Autodesk Inventor part; units mm, degrees
ref_plane "YZ Plane" through (0, 0, 0) normal (1, 0, 0) x (0, 1, 0)
ref_plane "XZ Plane" through (0, 0, 0) normal (0, 1, 0) x (-1, 0, 0)
ref_plane "XY Plane" through (0, 0, 0) normal (0, 0, 1) x (1, 0, 0)
sketch "Эскиз1" plane through (0, 0, 0) normal (0, 0, 1) x (1, 0, 0)
  line L0 (-12.2268, 10) -> (34.5444, 10)
  line L1 (-55.4556, 0) -> (49.5444, 0)
  line L2 (-12.2268, -10) -> (34.5444, -10)
  arc A0 (-15.534, 11.25) -> (-15.534, -11.25) centre (-25.4556, 0) ccw
  circle A1 centre (-25.4556, 0) radius 5
  line L3 (34.5444, 10) -> (34.5444, -10)
  arc A2 (-15.534, 11.25) -> (-12.2268, 10) centre (-12.2268, 15) ccw
  arc A3 (-12.2268, -10) -> (-15.534, -11.25) centre (-12.2268, -15) ccw
  point P0 (0, 0)
  point P1 (-14.2752, 10)
  point P2 (-14.2752, -10)
  dimension "d0" = 15
  dimension "d1" = 20
  dimension "d2" = 10
  dimension "d12" = 5
  dimension "d13" = 60
extrude "Выдавливание1" add sketch "Эскиз1" along normal blind 5 and the other way blind 5 contours L0 L3 L1 A1 A0 A2 | L3 L2 A3 A0 L1 A1
sketch "Эскиз4" plane through (0, 0, 0) normal (0, 0, 1) x (1, 0, 0)
  line L0 (-20.9089, 0) -> (125.4533, 0)
  line L1 (34.5444, 10) -> (34.5444, -10)
  line L2 (34.5444, 0) -> (114.5444, 0)
  line L3 (114.5444, 0) -> (114.5444, 20)
  line L4 (114.5444, 20) -> (34.5444, 20)
  line L5 (34.5444, 20) -> (34.5444, 0)
  point P0 (0, 0)
  dimension "d7" = 40
  dimension "d8" = 80
revolve "Вращение1" add sketch "Эскиз4" angle 360 about axis through (-10, 0, 0) along (1, 0, 0)
properties part number "поршень" material "Сталь"
Part model, mm, in its own coordinate system. A direction names the side the tool comes from. Give positions to 0.01 mm unless a question says otherwise; leave off trailing zeros. Loops run counter-clockwise (first coordinate to the right, second up) from the corner with the lowest first, then second, coordinate; pieces in that order, holes last. Notation, with made-up numbers: M 70,2 L 86,2 A28 ccw 86,30 Z; hole C 73,14.5 d4. An arc over 180 degrees is marked long. Return JSON: item names as keys, results as strings.
1) Saw through at B-B, the plane y = 0. List the corners of the cut face in (x, z), then the cut area to 3 significant figures.
Calculated:
{"outline": "M -40.46,-5 L -30.46,-5 L -30.46,5 L -40.46,5 Z; M -20.46,-5 L 34.54,-5 L 34.54,-20 L 114.54,-20 L 114.54,20 L 34.54,20 L 34.54,5 L -20.46,5 Z", "area": "3,850 mm2"}
2) Pull direction X, two halves, no side cores. Call faces 4 (the face through (-3, 0, 5)), 5 (the face through (-14.018, -10.332, -0.07)), 6 (the face through (114.544, 0, 0)): released by +X, released by -X, zero draft, split by the parting line, or undercut.
Calculated:
{"face 4": "zero draft", "face 5": "undercut", "face 6": "released by +X"}
3) Saw through at D-D, the plane y = 17. List the corners of the cut face in (x, z), then the cut area to 3 significant figures.
Calculated:
{"outline": "M 34.54,-10.54 L 114.54,-10.54 L 114.54,10.54 L 34.54,10.54 Z", "area": "1,690 mm2"}
4) Flat gauge pins, fed straight in: pin 1 Ø6 at (x, y) = (39, -4) entering from +Z (3 decimals); pin 2 Ø6 at (x, y) = (-25.46, 0) entering from -Z; pin 3 Ø3 at (x, z) = (7, 0) entering from -Y; pin 4 Ø6 at (y, z) = (6.5, 9.5) entering from -X. Where does each tip first touch, or does it go through?
Calculated:
{"pin 1": "stops at z = 19.975", "pin 2": "passes through", "pin 3": "stops at y = -10", "pin 4": "stops at x = 34.54"}
5) Saw through at C-C, the plane x = 19. List the corners of the cut face in (y, z).
Calculated:
{"outline": "M -10,-5 L 10,-5 L 10,5 L -10,5 Z"}
6) Saw through at A-A, the plane z = 0. List the corners of the cut face in (x, y), then the cut area to 3 significant figures.
Calculated:
{"outline": "M -15.53,-11.25 A5 cw -12.23,-10 L 34.54,-10 L 34.54,-20 L 114.54,-20 L 114.54,20 L 34.54,20 L 34.54,10 L -12.23,10 A5 cw -15.53,11.25 A15 ccw long Z; hole C -25.46,0 d10", "area": "4,750 mm2"}
7) 3-axis set-ups, long thin cutter, end or side, ignore diameter. For faces 1 (the face through (11, -10, 0)), 2 (the face through (-13.971, 10.314, -0.07)), 3 (the face through (-3, 0, -5)): which of +Z, -Z, +X, -X, +Y, -Y reach the whole face in a straight line?
Calculated:
{"face 1": "+Z, -Z, -Y", "face 2": "+Z, -Z, +Y", "face 3": "-Z, -X, +Y, -Y"}
8) Drill centre lines: line 1 (X direction, y = 0, z = -1); line 2 (Y direction, x = 14, z = -1); line 3 (X direction, y = -8, z = -8.5). Where is each one in solid material? Low to high.
Calculated:
{"line 1": "x = -40.46 to -30.46, -20.46 to 114.54", "line 2": "y = -10 to 10", "line 3": "x = 34.54 to 114.54"}
